Work out the finished part from the listing and answer in its coordinate system (mm). Face numbers are marked on the shaded views. A direction names the side the tool comes from. Round coordinates to 2 decimals unless told otherwise and drop trailing zeros. Order: outer loops, then holes, each group sorted by start corner. A loop starts at its lowest first (then second) coordinate and runs counter-clockwise, first axis right, second up. Notation, with made-up numbers: (15.25, -25) -> (23.25, -25) arc R9 cw to (23.25, -14) -> close; hole circle Ø5 at (85, 1). An arc over 180 degrees is marked (long way). Use a Markdown table: item, result. Add a question column.
Item 1: Find the intervals of material crossed by L1, parallel to Z at x = 20.45, y = -0.9; L2, parallel to X at y = -2.5, z = 18; L3, parallel to Y at x = 3, z = -5, in increasing order. Write a range as [from, to].
Item 2: A cutting plane is placed at C-C, the plane y = -5. Determine the outline of the cut face in (x, z).
Item 3: A cutting plane is placed at A-A, the plane z = -31.5. Determine the outline of the cut face in (x, y), plus the area to 3 significant figures.
Item 4: A tool of negligible diameter and unlimited length cuts with its end or side. For the marked faces 1, 2, 3 and 4, from which of +Z, -Z, +X, -X, +Y, -Y can it reach the whole face along a straight path? Write none if from no direction.
Item 5: For a pull along X with two mould halves and no side action, classify the marked faces 5 and 6 as +X half, -X half, draft (parallel to the pull), parting line (faces both ways), or undercut.
Item 6: A cutting plane is placed at D-D, the plane z = -4. Determine the outline of the cut face in (x, y), plus the area to 3 significant figures.
Item 7: A cutting plane is placed at B-B, the plane x = 20.45. Determine the outline of the cut face in (y, z).
Item 8: Flat-ended cylindrical pins translate along their axes: P1, Ø2, axis at x = -37, y = -4.5, coming from the -Z side; P2, Ø6, axis at x = 20.45, z = 31.5, coming from the -Y side; P3, Ø0.7, axis at y = -1, z = 32, coming from the -X side; P4, Ø4.5, axis at x = -20.45, z = -31.5, coming from the +Y side. Find the tip coordinate at first contact, or state that the pin passes through.
from build123d import *

# Parameters (mm, degrees)
F0_R     = 2.5
F1_DEPTH = 2.29
F0_W     = 24
F0_H     = 50
F2_DEPTH = 7


with BuildPart() as f1:
    # F0 (on Front) → F1 (new body)
    with BuildSketch(Plane.XZ):
        Polygon((-29.5, -38.5), (29.5, -38.5), (29.5, -24.384001), (29.5, 25.615999), (29.5, 38.5), (-29.5, 38.5), (-29.5, 25.615999), (-29.5, -24.384001), align=None)
        with Locations((-20.45, -31.5)):
            Circle(F0_R, mode=Mode.SUBTRACT)
        with Locations((20.45, -31.5)):
            Circle(F0_R, mode=Mode.SUBTRACT)
        with Locations((-20.45, 31.5)):
            Circle(F0_R, mode=Mode.SUBTRACT)
        with Locations((20.45, 31.5)):
            Circle(F0_R, mode=Mode.SUBTRACT)
    extrude(amount=F1_DEPTH)

    # F0 (on Front) → F2 (join)
    with BuildSketch(Plane.XZ):
        with Locations((41.5, 0.615999)):
            Rectangle(F0_W, F0_H)
        with Locations((-41.5, 0.615999)):
            Rectangle(F0_W, F0_H)
    extrude(amount=F2_DEPTH)


solid = f1.part
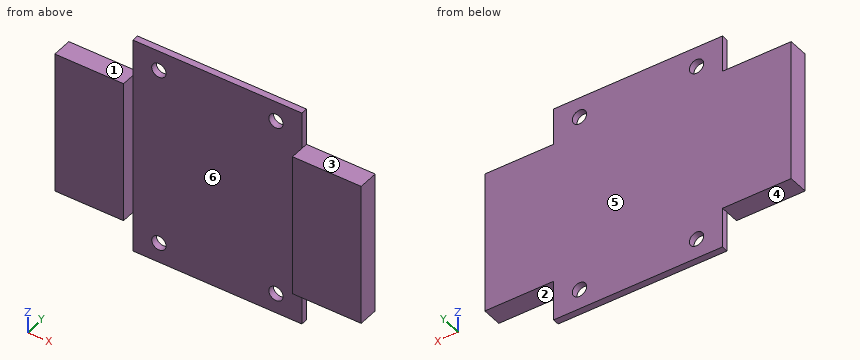
Reported:
| question | item | result |
|---|---|---|
| 1 | L1 | [-38.5, -34], [-29, 29], [34, 38.5] |
| 1 | L2 | [-53.5, -29.5], [29.5, 53.5] |
| 1 | L3 | [-2.29, 0] |
| 2 | outline | (-53.5, -24.38) -> (-29.5, -24.38) -> (-29.5, 25.62) -> (-53.5, 25.62) -> close; (29.5, -24.38) -> (53.5, -24.38) -> (53.5, 25.62) -> (29.5, 25.62) -> close |
| 3 | outline | (-29.5, -2.29) -> (-22.95, -2.29) -> (-22.95, 0) -> (-29.5, 0) -> close; (-17.95, -2.29) -> (17.95, -2.29) -> (17.95, 0) -> (-17.95, 0) -> close; (22.95, -2.29) -> (29.5, -2.29) -> (29.5, 0) -> (22.95, 0) -> close |
| 3 | area | 112 mm² |
| 4 | face 1 | +Z, -X, +Y, -Y |
| 4 | face 2 | -Z, +X, +Y, -Y |
| 4 | face 3 | +Z, +X, +Y, -Y |
| 4 | face 4 | -Z, -X, +Y, -Y |
| 5 | face 5 | draft |
| 5 | face 6 | undercut |
| 6 | outline | (-53.5, -7) -> (-29.5, -7) -> (-29.5, -2.29) -> (29.5, -2.29) -> (29.5, -7) -> (53.5, -7) -> (53.5, 0) -> (-53.5, 0) -> close |
| 6 | area | 471 mm² |
| 7 | outline | (-2.29, -38.5) -> (0, -38.5) -> (0, -34) -> (-2.29, -34) -> close; (-2.29, -29) -> (0, -29) -> (0, 29) -> (-2.29, 29) -> close; (-2.29, 34) -> (0, 34) -> (0, 38.5) -> (-2.29, 38.5) -> close |
| 8 | P1 | z = -24.38 |
| 8 | P2 | y = -2.29 |
| 8 | P3 | x = -29.5 |
| 8 | P4 | through |
